```python
from build123d import *

# Parameters (mm, degrees)
CROQUIS1_W                 = 19.8
CROQUIS1_H                 = 11.5
SALIENTE_EXTRUIR1_DEPTH    = 70.5
VACIADO1_T                 = -2
CROQUIS5_W                 = 15.8
CROQUIS5_H                 = 2
SALIENTE_EXTRUIR2_DEPTH    = 2
CROQUIS6_W                 = 19.8
CROQUIS6_H                 = 8
SALIENTE_EXTRUIR4_DEPTH    = 16
SALIENTE_EXTRUIR5_DEPTH    = 19.8
CROQUIS10_R                = 2
CORTAR_EXTRUIR4_DEPTH      = 19.8
CORTAR_EXTRUIR3_DEPTH      = 43.653516854
CORTAR_EXTRUIR3_DEPTH_BACK = 43.653516854
CROQUIS8_R                 = 1
CROQUIS11_W                = 15.8
CROQUIS11_H                = 26
CORTAR_EXTRUIR5_DEPTH      = 2
REDONDEO2_R                = 8
REDONDEO4_R                = 1
REDONDEO5_R                = 1
REDONDEO6_R                = 1
REDONDEO7_R                = 1
REDONDEO8_R                = 1


with BuildPart() as part:
    # Croquis1 → Saliente-Extruir1 (new body)
    with BuildSketch(Plane(origin=(0, 0, 0), x_dir=(0, 1, 0), z_dir=(0, 0, 1))):
        Rectangle(CROQUIS1_W, CROQUIS1_H)
    extrude(amount=SALIENTE_EXTRUIR1_DEPTH)

    # Vaciado1
    vaciado1_openings = [part.faces().sort_by_distance(p)[0] for p in [
        (0, 0, 70.5),
    ]]
    offset(amount=VACIADO1_T, openings=vaciado1_openings, kind=Kind.INTERSECTION)

    # Croquis5 → Saliente-Extruir2 (add)
    with BuildSketch(Plane.YZ.offset(5.75)):
        with Locations((0, 69.5)):
            Rectangle(CROQUIS5_W, CROQUIS5_H)
    extrude(amount=-SALIENTE_EXTRUIR2_DEPTH)

    # Croquis6 → Saliente-Extruir4 (add)
    with BuildSketch(Plane(origin=(-5.75, 0, 0), x_dir=(0, -1, 0), z_dir=(-1, 0, 0))):
        with Locations((0, 29)):
            Rectangle(CROQUIS6_W, CROQUIS6_H)
    extrude(amount=SALIENTE_EXTRUIR4_DEPTH)

    # Croquis9 → Saliente-Extruir5 (add)
    with BuildSketch(Plane.XZ.offset(9.9)):
        Polygon((-5.75, 70.5), (-12.75, 33), (-5.75, 33), align=None)
        Polygon((-5.75, 0), (-12.75, 25), (-5.75, 25), align=None)
    extrude(amount=-SALIENTE_EXTRUIR5_DEPTH)

    # Croquis10 → Cortar-Extruir4 (cut)
    with BuildSketch(Plane.XZ.offset(9.9)):
        with Locations(Location((-16.745253682, 29, 0), (0, 0, 270))):
            Circle(CROQUIS10_R)
    extrude(amount=-CORTAR_EXTRUIR4_DEPTH, mode=Mode.SUBTRACT)

    # Croquis8 → Cortar-Extruir3 (cut, two sides: drawn at the far end of the back side and taken through both)
    with BuildSketch(Plane(origin=(-4, 0, 33), x_dir=(1, 0, 0), z_dir=(0, 0, 1)).offset(-CORTAR_EXTRUIR3_DEPTH_BACK)):
        with Locations((-12.75, 5.1)):
            Circle(CROQUIS8_R)
        with Locations((-12.75, -4.9)):
            Circle(CROQUIS8_R)
    extrude(amount=CORTAR_EXTRUIR3_DEPTH + CORTAR_EXTRUIR3_DEPTH_BACK, mode=Mode.SUBTRACT)

    # Croquis11 → Cortar-Extruir5 (cut)
    with BuildSketch(Plane.YZ.offset(5.75)):
        with Locations((0, 15)):
            Rectangle(CROQUIS11_W, CROQUIS11_H)
    extrude(amount=-CORTAR_EXTRUIR5_DEPTH, mode=Mode.SUBTRACT)

    # Redondeo2
    # the kernel refuses this fillet: 8 mm, written as the material it adds along each edge
    with BuildSketch(Plane(origin=(5.75, -7.9, 28), x_dir=(0, 1, 0), z_dir=(-1, 0, 0)), Plane(origin=(5.75, 7.9, 28), x_dir=(0, 0, -1), z_dir=(-1, 0, 0))) as redondeo2_piece_1:
        with BuildLine():
            CenterArc((REDONDEO2_R, REDONDEO2_R), REDONDEO2_R, 180, 90)
            Line((0, REDONDEO2_R), (0, 0))
            Line((0, 0), (REDONDEO2_R, 0))
        make_face()
    extrude(amount=2)

    # Redondeo4
    redondeo4_edges = [part.edges().sort_by_distance(p)[0] for p in [
        (-12.75, 0, 33),
    ]]
    fillet(redondeo4_edges, radius=REDONDEO4_R)

    # Redondeo5
    redondeo5_edges = [part.edges().sort_by_distance(p)[0] for p in [
        (5.75, 0, 70.5),
        (-5.75, 0, 70.5),
    ]]
    fillet(redondeo5_edges, radius=REDONDEO5_R)

    # Redondeo6
    redondeo6_edges = [part.edges().sort_by_distance(p)[0] for p in [
        (-12.941660805, -9.9, 33.230748054),
        (-12.941660805, 9.9, 33.230748054),
        (-9.25, 9.9, 51.75),
        (-9.25, -9.9, 51.75),
        (-0.084696812, 9.9, 70.5),
        (5.75, 9.9, 34.75),
        (5.457106781, 9.9, 70.207106781),
        (-5.558339195, 9.9, 70.269251946),
        (-0.084696812, -9.9, 70.5),
        (5.75, -9.9, 34.75),
        (5.457106781, -9.9, 70.207106781),
        (-5.558339195, -9.9, 70.269251946),
        (-17.665303188, 9.9, 33),
        (-17.665303188, -9.9, 33),
    ]]
    fillet(redondeo6_edges, radius=REDONDEO6_R)

    # Redondeo7
    redondeo7_edges = [part.edges().sort_by_distance(p)[0] for p in [
        (-0.5, 9.9, 0),
        (5.75, 0, 0),
        (-0.5, -9.9, 0),
        (5.457106781, -9.607106781, 0),
        (5.457106781, 9.607106781, 0),
        (-21.75, 0, 25),
    ]]
    fillet(redondeo7_edges, radius=REDONDEO7_R)

    # Redondeo8
    redondeo8_edges = [part.edges().sort_by_distance(p)[0] for p in [
        (-21.75, 9.9, 29),
        (-21.75, 0, 33),
        (-21.75, -9.607106781, 32.707106781),
        (-21.75, 9.607106781, 32.707106781),
        (-21.75, -9.9, 29),
        (-16.75, -9.9, 25),
        (-21.457106781, -9.9, 25.292893219),
        (-16.75, 9.9, 25),
        (-21.457106781, 9.9, 25.292893219),
    ]]
    fillet(redondeo8_edges, radius=REDONDEO8_R)


solid = part.part
```
Geometry: final body of the model. Coordinates: model frame, mm. A direction names the side the tool comes from. Give positions to 0.01 mm unless a question says otherwise; leave off trailing zeros. Loops run counter-clockwise (first coordinate to the right, second up) from the corner with the lowest first, then second, coordinate; pieces in that order, holes last. Notation, with made-up numbers: (61.25, 19.25) -> (117.25, 19.25) arc R15 cw to (117.25, 43.25) -> close; hole circle Ø2 at (88.5, -26). An arc over 180 degrees is marked (long way). Return JSON: item names as keys, results as strings.
Item 1: Access query for faces 5 (the flat face through (-3.75, 0, 36)), 6 (the flat face through (1, 0, 2)), 7 (the flat face through (-21.75, 0, 29)). Directions: +Z, -Z, +X, -X, +Y, -Y. A direction counts if a zero-diameter tool reaches every point of the face in a straight line with its end or side. Return the directions, or none.
Filled in:
{"face 5": "+Z", "face 6": "+X", "face 7": "+Z, -Z, -X, +Y, -Y"}
Item 2: Line query: line 1 (X direction, y = 5.1, z = 31.9); line 2 (Y direction, x = -16.75, z = 31.3); line 3 (X direction, y = 0.5, z = 29). Output: solid intervals per line, ascending.
Filled in:
{"line 1": "-21.75 to -17.75, -15.75 to -3.75, 3.75 to 5.75", "line 2": "-9.9 to -5.9, -3.9 to 4.1, 6.1 to 9.9", "line 3": "-21.75 to -18.75, -14.75 to -3.75, 3.75 to 5.75"}
Item 3: Mould query, pull axis Z, two halves, no side actions, for faces 1 (the flat face through (-17, 0, 33)), 2 (the flat face through (-1, 0, 0)), 3 (the cylindrical face through (-16.29, -5.79, 31.85)), 4 (the cylindrical face through (4.76, -5.65, 25.56)). Classes: released by +Z, released by -Z, zero draft, split by the parting line, or undercut.
Filled in:
{"face 1": "released by +Z", "face 2": "released by -Z", "face 3": "zero draft", "face 4": "undercut"}
Item 4: Section D-D, the plane z = 13. Output: boundary loops of the cut face in (x, y), plus the area to 3 significant figures.
Filled in:
{"outline": "(-9.39, -9.9) -> (4.75, -9.9) arc R1 ccw to (5.75, -8.9) -> (5.75, -7.9) -> (-3.75, -7.9) -> (-3.75, 7.9) -> (5.75, 7.9) -> (5.75, 8.9) arc R1 ccw to (4.75, 9.9) -> (-9.39, 9.9) -> close", "area": "149 mm^2"}
Item 5: Pin query (flat end, axial travel): P1, Ø3, axis at x = 0.5, y = -3.5, coming from the +Z side; P2, Ø12, axis at x = -16, z = 19, coming from the -Y side; P3, Ø2.5, axis at x = -16.75, y = 5.1, coming from the +Z side; P4, Ø2.5, axis at x = -16.5, y = 0, coming from the -Z side. Return the tip coordinate at first contact, or that it passes through.
Filled in:
{"P1": "z = 2", "P2": "y = -9.9", "P3": "z = 33", "P4": "z = 25"}
Item 6: Section B-B, the plane y = 0.75. Output: boundary loops of the cut face in (x, z).
Filled in:
{"outline": "(-21.75, 26) arc R1 ccw to (-20.75, 25) -> (-12.75, 25) -> (-5.75, 0) -> (4.75, 0) arc R1 ccw to (5.75, 1) -> (5.75, 2) -> (-3.75, 2) -> (-3.75, 70.5) -> (-4.92, 70.5) arc R1 ccw to (-5.9, 69.68) -> (-12.6, 33.82) arc R1 cw to (-13.58, 33) -> (-20.75, 33) arc R1 ccw to (-21.75, 32) -> close; (3.75, 27.95) -> (5.75, 27.95) -> (5.75, 69.5) arc R1 ccw to (4.75, 70.5) -> (3.75, 70.5) -> close; hole circle Ø4 at (-16.75, 29)"}
Item 7: Section C-C, the plane x = -2.75. Output: boundary loops of the cut face in (y, z), plus the area to 3 significant figures.
Filled in:
{"outline": "(-9.9, 1) arc R1 ccw to (-8.9, 0) -> (8.9, 0) arc R1 ccw to (9.9, 1) -> (9.9, 69.5) arc R1 ccw to (8.9, 70.5) -> (7.9, 70.5) -> (7.9, 2) -> (-7.9, 2) -> (-7.9, 70.5) -> (-8.9, 70.5) arc R1 ccw to (-9.9, 69.5) -> close", "area": "313 mm^2"}
Item 8: Section A-A, the plane z = 29. Output: boundary loops of the cut face in (x, y), plus the area to 3 significant figures.
Filled in:
{"outline": "(-21.75, -8.9) arc R1 ccw to (-20.75, -9.9) -> (-18.75, -9.9) -> (-18.75, 9.9) -> (-20.75, 9.9) arc R1 ccw to (-21.75, 8.9) -> close; (-14.75, -9.9) -> (4.75, -9.9) arc R1 ccw to (5.75, -8.9) -> (5.75, 8.9) arc R1 ccw to (4.75, 9.9) -> (-14.75, 9.9) -> close; hole (-3.75, -7.9) -> (3.75, -7.9) -> (3.75, 7.9) -> (-3.75, 7.9) -> close", "area": "346 mm^2"}
